Read the model definition and answer for the solid it produces. Units are mm, in the model's axes. A direction names the side the tool comes from. Coordinates: 2 decimals unless noted, no trailing zeros. Order: outer loops, then holes, each group sorted by start corner. A loop starts at its lowest first (then second) coordinate and runs counter-clockwise, first axis right, second up. Notation, with made-up numbers: (40.5, 86) -> (47.5, 86) arc R16 cw to (47.5, 108) -> close; hole circle Ø1 at (50, 69). An arc over 180 degrees is marked (long way). Use CSV: the item, a comma, the result in double quotes.
```python
from build123d import *

# Parameters (mm, degrees)
CROQUIS1_W              = 20.8
CROQUIS1_H              = 20
SALIENTE_EXTRUIR1_DEPTH = 2
SALIENTE_EXTRUIR2_DEPTH = 11.8
SALIENTE_EXTRUIR3_DEPTH = 6.2
CORTAR_EXTRUIR1_REACH   = 16.6
CROQUIS4_R              = 1.6
CORTAR_EXTRUIR2_DEPTH   = 3


with BuildPart() as part:
    # Croquis1 → Saliente-Extruir1 (new body)
    with BuildSketch(Plane.XY):
        with Locations((10.4, -10)):
            Rectangle(CROQUIS1_W, CROQUIS1_H)
    extrude(amount=SALIENTE_EXTRUIR1_DEPTH)

    # Croquis2 → Saliente-Extruir2 (add)
    with BuildSketch(Plane.XY.offset(2)):
        with BuildLine():
            Line((8.2, -11.2), (8.2, -20))
            Line((8.2, -20), (20.8, -20))
            Line((20.8, -20), (20.8, 0))
            Line((20.8, 0), (0, 0))
            Line((0, 0), (0, -3))
            ThreePointArc((0, -3), (5.798275606, -5.401724394), (8.2, -11.2))
        make_face()
    extrude(amount=SALIENTE_EXTRUIR2_DEPTH)

    # Croquis3 → Saliente-Extruir3 (add)
    with BuildSketch(Plane.XY.offset(13.8)):
        with BuildLine():
            Line((14.6, -20), (14.6, 0))
            Line((14.6, 0), (0, 0))
            Line((0, 0), (0, -3))
            ThreePointArc((0, -3), (5.798275606, -5.401724394), (8.2, -11.2))
            Line((8.2, -11.2), (8.2, -20))
            Line((8.2, -20), (14.6, -20))
        make_face()
    extrude(amount=SALIENTE_EXTRUIR3_DEPTH)

    # Croquis4 → Cortar-Extruir1 (cut, up to next)
    with BuildSketch(Plane(origin=(14.6, 0, 0), x_dir=(0, 0, -1), z_dir=(1, 0, 0)), mode=Mode.PRIVATE) as cortar_extruir1_sk1:
        with Locations((-16.9, -16.2)):
            Circle(CROQUIS4_R)
    cortar_extruir1_tool1 = extrude(cortar_extruir1_sk1.sketch, amount=-CORTAR_EXTRUIR1_REACH, mode=Mode.PRIVATE) & part.part
    add(cortar_extruir1_tool1.solids().sort_by_distance((14.6, -16.2, 16.9))[0], mode=Mode.SUBTRACT)

    # Croquis5 → Cortar-Extruir2 (cut)
    with BuildSketch(Plane.ZY.offset(-8.2)):
        Polygon((16.9, -19.490896534), (19.75, -17.845448267), (19.75, -14.554551733), (16.9, -12.909103466), (14.05, -14.554551733), (14.05, -17.845448267), align=None)
    extrude(amount=-CORTAR_EXTRUIR2_DEPTH, mode=Mode.SUBTRACT)


solid = part.part
```
Item 1: The mould has two halves that part along Y. Classify faces 1 (the flat face through (11, 0, 10)), 2 (the flat face through (10, -8, 20)), 3 (the flat face through (10, -16, 14.05)): +Y half, -Y half, draft (parallel to the pull), parting line (faces both ways), or undercut.
Return value:
face 1,"+Y half"
face 2,"draft"
face 3,"undercut"
Item 2: A tool of negligible diameter and unlimited length cuts with its end or side. For faces 4 (the flat face through (14.6, -10, 17)), 5 (the flat face through (9.68, -13.74, 18.34)), 6 (the cylindrical face through (5.734, -5.338, 10.874)), from which of +Z, -Z, +X, -X, +Y, -Y can it reach the whole face along a straight path? Write none if from no direction.
Return value:
face 4,"+Z, +X, +Y, -Y"
face 5,"-X"
face 6,"+Z, -X, -Y"
Item 3: Find section A-A, the plane y = -16.2. Give the vertices of the cut face in (x, z), then the cut area to 3 significant figures.
Return value:
outline,"(0, 0) -> (20.8, 0) -> (20.8, 13.8) -> (14.6, 13.8) -> (14.6, 15.3) -> (11.2, 15.3) -> (11.2, 14.05) -> (8.2, 14.05) -> (8.2, 2) -> (0, 2) -> close; (8.2, 19.75) -> (11.2, 19.75) -> (11.2, 18.5) -> (14.6, 18.5) -> (14.6, 20) -> (8.2, 20) -> close"
area,"202 mm^2"
Item 4: Find section B-B, the plane z = 17.25. Give the vertices of the cut face in (x, y), then the cut area to 3 significant figures.
Return value:
outline,"(0, -3) arc R8.2 cw to (8.2, -11.2) -> (8.2, -13.11) -> (11.2, -13.11) -> (11.2, -14.64) -> (14.6, -14.64) -> (14.6, 0) -> (0, 0) -> close; (8.2, -20) -> (14.6, -20) -> (14.6, -17.76) -> (11.2, -17.76) -> (11.2, -19.29) -> (8.2, -19.29) -> close"
area,"138 mm^2"
Item 5: Each of these flat-tipped pins is pushed along its axis until it touches: P1, Ø4.5, axis at y = -14.5, z = 15.5, coming from the -X side; P2, Ø4, axis at x = 3.5, y = -11, coming from the +Z side; P3, Ø5, axis at y = -16.2, z = 16.9, coming from the +X side. Where does it stop, or does it pass through?
Return value:
P1,"stops at x = 8.2"
P2,"stops at z = 2"
P3,"stops at x = 14.6"
Item 6: Find section D-D, the plane y = -9.75. Give the vertices of the cut face in (x, z), then the cut area to 3 significant figures.
Return value:
outline,"(0, 0) -> (20.8, 0) -> (20.8, 13.8) -> (14.6, 13.8) -> (14.6, 20) -> (8.07, 20) -> (8.07, 2) -> (0, 2) -> close"
area,"232 mm^2"
Item 7: Find section C-C, the plane x = 13.5. Give the vertices of the cut face in (y, z), then the cut area to 3 significant figures.
Return value:
outline,"(-20, 0) -> (0, 0) -> (0, 20) -> (-20, 20) -> close; hole circle Ø3.2 at (-16.2, 16.9)"
area,"392 mm^2"
Item 8: Straight lines are drawn through the part: line 1 along Y through (x, z) = (13.75, 16.9); line 2 along Z through (x, y) = (1.75, -13.5); line 3 along Z through (x, y) = (17.5, -9). For each, find the intervals that lie inside material, in ascending order.
Return value:
line 1,"y = -20 to -17.8, -14.6 to 0"
line 2,"z = 0 to 2"
line 3,"z = 0 to 13.8"
